Source: CAD feature listing. Evaluate the final solid. Frame: model axes, mm. A direction names the side the tool comes from. Give positions to 0.01 mm unless a question says otherwise; leave off trailing zeros. Order: outer loops, then holes, each group sorted by start corner. A loop starts at its lowest first (then second) coordinate and runs counter-clockwise, first axis right, second up. Notation, with made-up numbers: M 50,55.25 L 77,55.25 A12 ccw 77,70.25 Z; hole C 13.5,62.25 d5. An arc over 180 degrees is marked long. Answer as a JSON object with one key per item and string values. Group by question number.
1. Section query B-B (y = 0). Count the separate pieces of the cut face and the enclosed holes in it, plus the area to 3 significant figures.
2. Material intervals for L1, parallel to X at y = 0.5, z = 16; L2, parallel to Z at x = 38, y = 3.25; L3, parallel to X at y = 2.5, z = 18, sorted ascending. Write a range as [from, to].
3. Section query A-A (z = 29.5). Output: boundary loops of the cut face in (x, y).
4. Pin query (flat end, axial travel): P1, Ø1, axis at x = 56, y = 0, coming from the +Z side; P2, Ø1.1, axis at x = 56, z = 0.5, coming from the +Y side; P3, Ø1.6, axis at x = 44, y = 1.5, coming from the -Z side; P4, Ø0.5, axis at x = 72.5, z = 0.5, coming from the +Y side. Return the tip coordinate at first contact, or that it passes through.
5. Set-up query: faces 3 (the flat face through (97, 1, 17)), 4 (the flat face through (16, 1, 1)), 5 (the flat face through (60, 1, 34)), 6 (the flat face through (31.1, -2, 16)). Return all of +Z, -Z, +X, -X, +Y, -Y with unobstructed straight access to the full face (end or side cutting, diameter ignored); none if empty.
6. Pull-direction query (X, two-part tool) for faces 1 (the flat face through (28, 1, 1)), 2 (the flat face through (84, 1, 1)); classes: +X half, -X half, draft (parallel to the pull), parting line (faces both ways), or undercut.
7. Section query C-C (x = 54). Output: boundary loops of the cut face in (y, z), plus the area to 3 significant figures.
from build123d import *

# Parameters (mm, degrees)
F0_W      = 100
F0_H      = 35
F1_DEPTH  = 4
F2_T      = -3
F3_W      = 1
F3_H      = 35
F4_DEPTH  = 6
F5_W      = 2
F5_H      = 1
F6_DEPTH  = 6
F7_W      = 2.1
F7_H      = 3.1
F8_DEPTH  = 3
F9_W      = 6
F9_H      = 6
F9_W_2    = 2.1
F9_H_2    = 3.1
F10_DEPTH = 2


with BuildPart() as f1:
    # F0 (on Front) → F1 (new body, symmetric)
    with BuildSketch(Plane.XZ):
        with Locations((50, 17.5)):
            Rectangle(F0_W, F0_H)
    extrude(amount=F1_DEPTH, both=True)

    # F2
    f2_openings = [f1.faces().sort_by_distance(p)[0] for p in [
        (50, 4, 17.5),
    ]]
    offset(amount=F2_T, openings=f2_openings)

    # F3 (on face) → F4 (cut)
    with BuildSketch(Plane(origin=(0, 4, 0), x_dir=(-1, 0, 0), z_dir=(0, 1, 0))):
        with Locations((-99.5, 17.5)):
            Rectangle(F3_W, F3_H)
        with Locations((-0.5, 17.5)):
            Rectangle(F3_W, F3_H)
    extrude(amount=-F4_DEPTH, mode=Mode.SUBTRACT)

    # F5 (on face) → F6 (cut)
    with BuildSketch(Plane(origin=(0, 4, 0), x_dir=(-1, 0, 0), z_dir=(0, 1, 0))):
        with Locations((-96, 34.5)):
            Rectangle(F5_W, F5_H)
        with Locations((-96, 0.5)):
            Rectangle(F5_W, F5_H)
        with Locations((-92, 34.5)):
            Rectangle(F5_W, F5_H)
        with Locations((-92, 0.5)):
            Rectangle(F5_W, F5_H)
        with Locations((-88, 34.5)):
            Rectangle(F5_W, F5_H)
        with Locations((-88, 0.5)):
            Rectangle(F5_W, F5_H)
        with Locations((-84, 34.5)):
            Rectangle(F5_W, F5_H)
        with Locations((-84, 0.5)):
            Rectangle(F5_W, F5_H)
        with Locations((-80, 34.5)):
            Rectangle(F5_W, F5_H)
        with Locations((-80, 0.5)):
            Rectangle(F5_W, F5_H)
        with Locations((-76, 34.5)):
            Rectangle(F5_W, F5_H)
        with Locations((-76, 0.5)):
            Rectangle(F5_W, F5_H)
        with Locations((-72, 34.5)):
            Rectangle(F5_W, F5_H)
        with Locations((-72, 0.5)):
            Rectangle(F5_W, F5_H)
        with Locations((-68, 34.5)):
            Rectangle(F5_W, F5_H)
        with Locations((-68, 0.5)):
            Rectangle(F5_W, F5_H)
        with Locations((-64, 34.5)):
            Rectangle(F5_W, F5_H)
        with Locations((-64, 0.5)):
            Rectangle(F5_W, F5_H)
        with Locations((-60, 34.5)):
            Rectangle(F5_W, F5_H)
        with Locations((-60, 0.5)):
            Rectangle(F5_W, F5_H)
        with Locations((-56, 34.5)):
            Rectangle(F5_W, F5_H)
        with Locations((-56, 0.5)):
            Rectangle(F5_W, F5_H)
        with Locations((-52, 34.5)):
            Rectangle(F5_W, F5_H)
        with Locations((-52, 0.5)):
            Rectangle(F5_W, F5_H)
        with Locations((-48, 34.5)):
            Rectangle(F5_W, F5_H)
        with Locations((-48, 0.5)):
            Rectangle(F5_W, F5_H)
        with Locations((-44, 34.5)):
            Rectangle(F5_W, F5_H)
        with Locations((-44, 0.5)):
            Rectangle(F5_W, F5_H)
        with Locations((-40, 34.5)):
            Rectangle(F5_W, F5_H)
        with Locations((-40, 0.5)):
            Rectangle(F5_W, F5_H)
        with Locations((-36, 34.5)):
            Rectangle(F5_W, F5_H)
        with Locations((-36, 0.5)):
            Rectangle(F5_W, F5_H)
        with Locations((-32, 34.5)):
            Rectangle(F5_W, F5_H)
        with Locations((-32, 0.5)):
            Rectangle(F5_W, F5_H)
        with Locations((-28, 34.5)):
            Rectangle(F5_W, F5_H)
        with Locations((-28, 0.5)):
            Rectangle(F5_W, F5_H)
        with Locations((-24, 34.5)):
            Rectangle(F5_W, F5_H)
        with Locations((-24, 0.5)):
            Rectangle(F5_W, F5_H)
        with Locations((-20, 34.5)):
            Rectangle(F5_W, F5_H)
        with Locations((-20, 0.5)):
            Rectangle(F5_W, F5_H)
        with Locations((-16, 34.5)):
            Rectangle(F5_W, F5_H)
        with Locations((-16, 0.5)):
            Rectangle(F5_W, F5_H)
        with Locations((-12, 34.5)):
            Rectangle(F5_W, F5_H)
        with Locations((-12, 0.5)):
            Rectangle(F5_W, F5_H)
        with Locations((-8, 34.5)):
            Rectangle(F5_W, F5_H)
        with Locations((-8, 0.5)):
            Rectangle(F5_W, F5_H)
        with Locations((-4, 34.5)):
            Rectangle(F5_W, F5_H)
        with Locations((-4, 0.5)):
            Rectangle(F5_W, F5_H)
    extrude(amount=-F6_DEPTH, mode=Mode.SUBTRACT)

    # F7 (on face) → F8 (cut)
    with BuildSketch(Plane.XZ.offset(4)):
        with Locations((67.65, 15.95)):
            Rectangle(F7_W, F7_H)
        with Locations((30.05, 15.95)):
            Rectangle(F7_W, F7_H)
    extrude(amount=-F8_DEPTH, mode=Mode.SUBTRACT)

    # F9 (on face) → F10 (join)
    with BuildSketch(Plane(origin=(0, -1, 0), x_dir=(-1, 0, 0), z_dir=(0, 1, 0))):
        with Locations((-68.1, 15.4)):
            Rectangle(F9_W, F9_H)
        with Locations((-67.65, 15.95)):
            Rectangle(F9_W_2, F9_H_2, mode=Mode.SUBTRACT)
        with Locations((-30.5, 15.4)):
            Rectangle(F9_W, F9_H)
        with Locations((-30.05, 15.95)):
            Rectangle(F9_W_2, F9_H_2, mode=Mode.SUBTRACT)
    extrude(amount=F10_DEPTH)


solid = f1.part
Answer sheet:
{
 "1": {"separate pieces": "3", "enclosed holes": "3", "area": "667 mm^2"},
 "2": {"L1": "[1, 3], [27.5, 29], [31.1, 33.5], [65.1, 66.6], [68.7, 71.1], [97, 99]", "L2": "[0, 3], [32, 35]", "L3": "[1, 3], [97, 99]"},
 "3": {"outline": "M 0,-4 L 100,-4 L 100,-2 L 99,-2 L 99,4 L 97,4 L 97,-1 L 3,-1 L 3,4 L 1,4 L 1,-2 L 0,-2 Z"},
 "4": {"P1": "z = 34", "P2": "y = 4", "P3": "z = 1", "P4": "y = -2"},
 "5": {"face 3": "+Y", "face 4": "-Z, +Y", "face 5": "+Z, +Y", "face 6": "+Y, -Y"},
 "6": {"face 1": "undercut", "face 2": "undercut"},
 "7": {"outline": "M -4,0 L 4,0 L 4,3 L -1,3 L -1,32 L 4,32 L 4,35 L -4,35 Z", "area": "135 mm^2"}
}
